The listing builds one solid part. Answer for the finished solid, in the listing's coordinates (mm). A direction names the side the tool comes from. Coordinates: 2 decimals unless noted, no trailing zeros. Loops run counter-clockwise (first coordinate to the right, second up) from the corner with the lowest first, then second, coordinate; pieces in that order, holes last. Notation, with made-up numbers: (-37.75, 34) - (-21.75, 34) arc R10 cw to (-21.75, 49) - close; hole circle Ø4 at (43, -34.75). An arc over 180 degrees is marked (long way). Write each question's results on one line, items separated by ' | '. Start each with the question number.
(1) Find section A-A on y = 119.5. Determine the outline of the cut face in (x, z).
(2) For faces 1 (the flat face through (-7.6, 7.5, -7.6)), 2 (the flat face through (5.25, 69, -12)), 3 (the flat face through (8.651, 20, -14)), 4 (the flat face through (-4.4, 0, -4.4)), 5 (the cylindrical face through (8.2, 7.6, -0.08)), determine the directions among +Z, -Z, +X, -X, +Y, -Y from which every point of the face is accessible in a straight line to the end or side of a thin tool.
(3) Determine the mould class of faces 6 (the cylindrical face through (-8.588, 6.116, -12.352)), 7 (the flat face through (9.7, 69.2, -7.3)), 8 (the flat face through (8, 125, -12)) for opening direction Z: released by +Z, released by -Z, zero draft, split by the parting line, or undercut.
(4) Find section B-B on y = 8. Determine the outline of the cut face in (x, z).
(5) Consider line 1 (Y direction, x = 6, z = -12); line 2 (X direction, y = 11, z = 0); line 3 (Y direction, x = 9, z = -3). Determine where each line is inside the solid, lowest interval first. Write a range as from..to.
(6) Given pin 1 Ø5 at (x, y) = (4.5, 98.5) entering from -Z; pin 2 Ø3.5 at (y, z) = (68, -11.5) entering from -X; pin 3 Ø3.5 at (y, z) = (21.5, -11) entering from +X, each flat-ended and moving along its own axis, determine where each tip first touches the part or whether it passes through.
(7) Find section C-C on y = 37.5. Determine the outline of the cut face in (x, z).
from build123d import *

# Parameters (mm, degrees)
SKIZZE1_R                        = 18.75
AUFSATZ_LINEAR_AUSTRAGEN1_DEPTH  = 15
SKIZZE2_R                        = 1.8
SKIZZE2_R_2                      = 1.65
SCHNITT_LINEAR_AUSTRAGEN1_DEPTH  = 16
AUFSATZ_LINEAR_AUSTRAGEN2_DEPTH  = 110
SKIZZE10_R                       = 3
SCHNITT_LINEAR_AUSTRAGEN5_DEPTH  = 8
KREISMUSTER1_COUNT               = 4
SKIZZE11_R                       = 1.6
SCHNITT_LINEAR_AUSTRAGEN6_DEPTH  = 14.5000001
SKIZZE16_R                       = 3.5
SCHNITT_LINEAR_AUSTRAGEN10_DEPTH = 2.1
SCHNITT_LINEAR_AUSTRAGEN11_DEPTH = 126.0000001


with BuildPart() as part:
    # Skizze1 → Aufsatz-Linear austragen1 (new body)
    with BuildSketch(Plane(origin=(0, 0, 0), x_dir=(1, 0, 0), z_dir=(0, 1, 0))):
        Circle(SKIZZE1_R)
    extrude(amount=AUFSATZ_LINEAR_AUSTRAGEN1_DEPTH)

    # Skizze2 → Schnitt-Linear austragen1 (cut, through all)
    with BuildSketch(Plane(origin=(0, 15, 0), x_dir=(1, 0, 0), z_dir=(0, 1, 0))):
        with Locations((0, 10)):
            Circle(SKIZZE2_R)
        with Locations((10, 0)):
            Circle(SKIZZE2_R)
        with Locations((0, -10)):
            Circle(SKIZZE2_R)
        with Locations((-10, 0)):
            Circle(SKIZZE2_R)
        Circle(SKIZZE2_R_2)
    extrude(amount=-SCHNITT_LINEAR_AUSTRAGEN1_DEPTH, mode=Mode.SUBTRACT)

    # Skizze4 → Aufsatz-Linear austragen2 (add)
    with BuildSketch(Plane(origin=(0, 15, 0), x_dir=(1, 0, 0), z_dir=(0, 1, 0))):
        with BuildLine():
            Line((5.25, 17), (5.25, 6))
            Line((5.25, 6), (8.607298894, 6))
            Line((8.607298894, 6), (10.750900369, 8.554644759))
            Line((10.750900369, 8.554644759), (10.750900369, 15.361661409))
            ThreePointArc((10.750900369, 15.361661409), (8.108477711, 16.906066639), (5.25, 18))
            Line((5.25, 18), (5.25, 17))
        make_face()
    extrude(amount=AUFSATZ_LINEAR_AUSTRAGEN2_DEPTH)

    # Skizze10 → Schnitt-Linear austragen5 (cut)
    with BuildSketch(Plane(origin=(13.258252147, 0, 13.258252147), x_dir=(0, -1, 0), z_dir=(0.707106781, 0, 0.707106781))):
        with Locations((-7.5, 0)):
            Circle(SKIZZE10_R)
    schnitt_linear_austragen5 = extrude(amount=-SCHNITT_LINEAR_AUSTRAGEN5_DEPTH, mode=Mode.SUBTRACT)

    # Kreismuster1: Schnitt-Linear austragen5 ×4 about axis
    kreismuster1_axis = Axis((0, 0, 0), (0, 1, 0))
    for i in range(1, KREISMUSTER1_COUNT):
        add(schnitt_linear_austragen5.rotate(kreismuster1_axis, i * 360 / KREISMUSTER1_COUNT), mode=Mode.SUBTRACT)

    # Skizze11 → Schnitt-Linear austragen6 (cut, through all)
    with BuildSketch(Plane.ZY.offset(-5.25)):
        with Locations((-12.5, 119.5)):
            Circle(SKIZZE11_R)
        with Locations((-12.5, 21)):
            Circle(SKIZZE11_R)
    extrude(amount=-SCHNITT_LINEAR_AUSTRAGEN6_DEPTH, mode=Mode.SUBTRACT)

    # Skizze16 → Schnitt-Linear austragen10 (cut)
    with BuildSketch(Plane(origin=(10.750900369, 0, 0), x_dir=(0, 0, -1), z_dir=(1, 0, 0))):
        with Locations((12.5, 119.5)):
            Circle(SKIZZE16_R)
        with Locations((12.5, 21)):
            Circle(SKIZZE16_R)
    extrude(amount=-SCHNITT_LINEAR_AUSTRAGEN10_DEPTH, mode=Mode.SUBTRACT)

    # Skizze17 → Schnitt-Linear austragen11 (cut, through all)
    with BuildSketch(Plane(origin=(0, 125, 0), x_dir=(1, 0, 0), z_dir=(0, 1, 0))):
        with BuildLine():
            Line((5.25, 18), (10.750900369, 15.361661409))
            ThreePointArc((10.750900369, 15.361661409), (8.108477711, 16.906066639), (5.25, 18))
        make_face()
    extrude(amount=-SCHNITT_LINEAR_AUSTRAGEN11_DEPTH, mode=Mode.SUBTRACT)

    # Skizze18 → Schnitt-Rotation1 (revolve, cut)
    with BuildSketch(Plane.XY):
        Polygon((0, 0), (6, 0), (7.2, 15), (0, 15), align=None)
    revolve(axis=Axis((0, 15, 0), (0, -1, 0)), mode=Mode.SUBTRACT)


solid = part.part
Values:
1) outline: (5.25, -18) - (9.42, -16) - (8.65, -16) - (8.65, -14.1) - (5.25, -14.1) - close; (5.25, -10.9) - (8.65, -10.9) - (8.65, -9) - (10.75, -9) - (10.75, -8.55) - (8.61, -6) - (5.25, -6) - close
2) face 1: none | face 2: +Z, -Z, -X, +Y | face 3: +X | face 4: +Z, -Z, +X, -X, -Y | face 5: +Y, -Y
3) face 6: undercut | face 7: released by +Z | face 8: zero draft
4) outline: (-15.18, -11) - (-9.69, -5.51) - (-5.51, -9.69) - (-11, -15.18) arc R18.75 ccw to (5.25, -18) - (10.75, -15.36) arc R18.75 ccw to (11, -15.18) - (5.51, -9.69) - (9.69, -5.51) - (15.18, -11) arc R18.75 ccw to (15.18, 11) - (9.69, 5.51) - (5.51, 9.69) - (11, 15.18) arc R18.75 ccw to (-11, 15.18) - (-5.51, 9.69) - (-9.69, 5.51) - (-15.18, 11) arc R18.75 ccw to start; hole circle Ø3.6 at (-10, 0); hole circle Ø13.28 at (0, 0); hole circle Ø3.6 at (0, -10); hole circle Ø3.6 at (0, 10); hole circle Ø3.6 at (10, 0)
5) line 1: y = 0..19.48, 22.52..117.98, 121.02..125 | line 2: x = -18.75..-11.8, -8.2..-6.88, 6.88..8.2, 11.8..18.75 | line 3: y = 0..15
6) pin 1: stops at z = -18 | pin 2: stops at x = 5.25 | pin 3: stops at x = 8.65
7) outline: (5.25, -18) - (10.75, -15.36) - (10.75, -8.55) - (8.61, -6) - (5.25, -6) - close
